```python
from build123d import *

# Parameters (mm, degrees)
SKETCH1_R           = 30
SKETCH1_R_2         = 7
BOSS_EXTRUDE1_DEPTH = 10
FILLET1_R           = 15
FILLET2_R           = 25
CUT_EXTRUDE1_DEPTH  = 21


with BuildPart() as part:
    # Sketch1 → Boss-Extrude1 (new body, symmetric)
    with BuildSketch(Plane(origin=(0, 0, 0), x_dir=(1, 0, 0), z_dir=(0, 1, 0))):
        with BuildLine():
            Line((27.935473676, 25.760615491), (128.063755469, 9.084385863))
            ThreePointArc((128.063755469, 9.084385863), (155, 0), (128.063755469, -9.084385863))
            Line((128.063755469, -9.084385863), (27.935473676, -25.760615491))
            ThreePointArc((27.935473676, -25.760615491), (-38, 0), (27.935473676, 25.760615491))
        make_face()
        Circle(SKETCH1_R, mode=Mode.SUBTRACT)
        with Locations((140, 0)):
            Circle(SKETCH1_R_2, mode=Mode.SUBTRACT)
    extrude(amount=BOSS_EXTRUDE1_DEPTH, both=True)

    # Fillet1
    fillet1_edges = [part.edges().sort_by_distance(p)[0] for p in [
        (128.063755469, 0, -9.084385863),
        (128.063755469, 0, 9.084385863),
    ]]
    fillet(fillet1_edges, radius=FILLET1_R)

    # Fillet2
    fillet2_edges = [part.edges().sort_by_distance(p)[0] for p in [
        (27.935473676, 0, -25.760615491),
        (27.935473676, 0, 25.760615491),
    ]]
    fillet(fillet2_edges, radius=FILLET2_R)

    # Sketch2 → Cut-Extrude1 (cut, through all)
    with BuildSketch(Plane.XZ.offset(10)):
        with BuildLine():
            Line((42.299222529, 16.271932074), (113.347981366, 4.438857582))
            ThreePointArc((113.347981366, 4.438857582), (117.108695652, 0), (113.347981366, -4.438857582))
            Line((113.347981366, -4.438857582), (42.299222529, -16.271932074))
            ThreePointArc((42.299222529, -16.271932074), (37.766889928, -14.690866644), (36.65479466, -10.021278781))
            ThreePointArc((36.65479466, -10.021278781), (38, 0), (36.65479466, 10.021278781))
            ThreePointArc((36.65479466, 10.021278781), (37.766889928, 14.690866644), (42.299222529, 16.271932074))
        make_face()
    extrude(amount=-CUT_EXTRUDE1_DEPTH, mode=Mode.SUBTRACT)


solid = part.part
```
The listing builds one solid part. Answer for the finished solid, in the listing's coordinates (mm). A direction names the side the tool comes from. Coordinates: 2 decimals unless noted, no trailing zeros. Order: outer loops, then holes, each group sorted by start corner. A loop starts at its lowest first (then second) coordinate and runs counter-clockwise, first axis right, second up. Notation, with made-up numbers: M 24,71.5 L 63,71.5 A34 ccw 63,103.5 Z; hole C 12,-35.75 d6. An arc over 180 degrees is marked long. Answer as a JSON object with one key per item and string values. Group by question number.
1. Straight lines are drawn through the part: line 1 (X direction, y = 2, z = 0.5); line 2 (Z direction, x = 0, y = -4); line 3 (X direction, y = 1.5, z = -2). For each, find the intervals that lie inside material, in ascending order.
2. Section C-C on y = -5.25 is taken. Write down the section's boundary in (x, z).
3. Section D-D on x = 79 is taken. Write down the section's boundary in (y, z).
4. Section B-B on x = 0 is taken. Write down the section's boundary in (y, z).
5. Section A-A on z = 0 is taken. Write down the section's boundary in (x, y), then the cut area to 3 significant figures.
6. Flat-ended cylindrical pins translate along their axes: P1, Ø6, axis at x = 58, y = 4, coming from the +Z side; P2, Ø12, axis at x = 3, y = 0, coming from the +Z side; P3, Ø12, axis at x = 31.5, y = 4, coming from the +Z side. Find the tip coordinate at first contact, or state that the pin passes through.
7. A tool of negligible diameter and unlimited length cuts with its end or side. For faces 5 (the cylindrical face through (38, 0, 0)), 6 (the flat face through (59, 10, -14)), 7 (the flat face through (78.73, 0.14, 17.3)), 8 (the flat face through (77.53, 0.14, -17.5)), 9 (the flat face through (59, -10, -14)), from which of +Z, -Z, +X, -X, +Y, -Y can it reach the whole face along a straight path? Write none if from no direction.
8. Determine the mould class of faces 1 (the cylindrical face through (29.1, 0.1, 26.4)), 2 (the cylindrical face through (-37.98, 0.14, 1.19)), 3 (the cylindrical face through (-29.97, -0.14, -1.32)), 4 (the cylindrical face through (37.72, -0.14, 14.64)) for opening direction X: released by +X, released by -X, zero draft, split by the parting line, or undercut.
Values follow:
{
 "1": {"line 1": "-38 to -30, 30 to 38, 117.08 to 133.02, 146.98 to 154.99", "line 2": "-38 to -30, 30 to 38", "line 3": "-37.95 to -29.93, 29.93 to 37.95, 116.64 to 133.29, 146.71 to 154.87"},
 "2": {"outline": "M 23.73,-29.68 A25 cw 35.24,-24.54 L 121.03,-10.26 A15 cw 131.75,-12.53 A15 ccw long 131.75,12.53 A15 cw 121.03,10.26 L 35.24,24.54 A25 cw 23.73,29.68 A38 ccw long Z; hole C 0,0 d60; hole M 36.65,-10.02 A5 ccw 42.3,-16.27 L 113.35,-4.44 A4.5 ccw 113.35,4.44 L 42.3,16.27 A5 ccw 36.65,10.02 A38 cw Z; hole C 140,0 d14"},
 "3": {"outline": "M -10,-17.26 L 10,-17.26 L 10,-10.16 L -10,-10.16 Z; M -10,10.16 L 10,10.16 L 10,17.26 L -10,17.26 Z"},
 "4": {"outline": "M -10,-38 L 10,-38 L 10,-30 L -10,-30 Z; M -10,30 L 10,30 L 10,38 L -10,38 Z"},
 "5": {"outline": "M -38,-10 L -30,-10 L -30,10 L -38,10 Z; M 30,-10 L 38,-10 L 38,10 L 30,10 Z; M 117.11,-10 L 133,-10 L 133,10 L 117.11,10 Z; M 147,-10 L 155,-10 L 155,10 L 147,10 Z", "area": "798 mm2"},
 "6": {"P1": "z = 21.25", "P2": "z = 38", "P3": "z = 28.39"},
 "7": {"face 5": "+Y, -Y", "face 6": "+Z, -Z, +X, -X, +Y", "face 7": "+Z, +Y, -Y", "face 8": "-Z, +Y, -Y", "face 9": "+Z, -Z, +X, -X, -Y"},
 "8": {"face 1": "released by +X", "face 2": "split by the parting line", "face 3": "undercut", "face 4": "undercut"}
}
